Part model, mm, in its own coordinate system. A direction names the side the tool comes from. Give positions to 0.01 mm unless a question says otherwise; leave off trailing zeros. Write each loop counter-clockwise with the first axis right and the second up, starting at its lowest first coordinate (ties: lowest second). Pieces come first, ordered by that corner, then holes. Notation, with made-up numbers: M -25,67.25 L 0,67.25 A22 ccw 0,74.25 Z; hole C 67.5,67.5 d7. An arc over 180 degrees is marked long. Use a Markdown table: item, result. Add a question column.
from build123d import *

# Parameters (mm, degrees)
SKETCH_1_R                = 77.5
EXTRUDE_1_DEPTH           = 35
SKETCH_2_R                = 15
CUT_EXTRUDE_1_DEPTH       = 116.05433499
CHAMFER_1_SIZE            = 1
HOLE_WIZARD_1_D           = 8
HOLE_WIZARD_1_CBORE_D     = 14
HOLE_WIZARD_1_CBORE_DEPTH = 9
PATTERN_CIRCULAR_1_COUNT  = 5
HOLE_WIZARD_M8_1_D        = 6.8
CUT_EXTRUDE_2_DEPTH       = 24
FILLET_1_R                = 5


with BuildPart() as part:
    # 草图1 → 凸台-拉伸1 (new body)
    with BuildSketch(Plane.XY):
        Circle(SKETCH_1_R)
    extrude(amount=EXTRUDE_1_DEPTH)

    # 草图2 → 切除-拉伸1 (cut, through all)
    with BuildSketch(Plane.XY.offset(35)):
        with Locations((-4, -57)):
            Circle(SKETCH_2_R)
    extrude(amount=-CUT_EXTRUDE_1_DEPTH, mode=Mode.SUBTRACT)

    # 倒角1
    chamfer_1_edges = [part.edges().sort_by_distance(p)[0] for p in [
        (-19, -57, 0),
        (-19, -57, 35),
    ]]
    chamfer(chamfer_1_edges, length=CHAMFER_1_SIZE)

    # 孔1 (through all)
    with Locations(Plane(origin=(0, 0, 0), x_dir=(1, 0, 0), z_dir=(0, 0, -1))):
        with Locations((0, -70)):
            hole_wizard_1 = CounterBoreHole(HOLE_WIZARD_1_D / 2, HOLE_WIZARD_1_CBORE_D / 2, HOLE_WIZARD_1_CBORE_DEPTH)

    # 阵列(圆周)1: 孔1 ×5 about axis
    pattern_circular_1_axis = Axis((0, 0, 0), (0, 0, 1))
    for i in range(1, PATTERN_CIRCULAR_1_COUNT):
        add(hole_wizard_1.rotate(pattern_circular_1_axis, i * 360 / PATTERN_CIRCULAR_1_COUNT), mode=Mode.SUBTRACT)

    # M8 螺纹孔1 (through all)
    with Locations(Plane.XY.offset(35)):
        with Locations((-56.631189606, 41.14496766), (56.631189606, -41.14496766)):
            Hole(HOLE_WIZARD_M8_1_D / 2)

    # 草图7 → 切除-拉伸2 (cut)
    with BuildSketch(Plane.XY.offset(35)):
        with BuildLine():
            ThreePointArc((57.446485936, 30.412189227), (38.206041399, 52.586104634), (11.171770317, 64.032738095))
            ThreePointArc((11.171770317, 64.032738095), (8.869948511, 63.894555935), (6.87493558, 62.738095238))
            ThreePointArc((6.87493558, 62.738095238), (0, 60), (-6.87493558, 62.738095238))
            ThreePointArc((-6.87493558, 62.738095238), (-8.869948511, 63.894555935), (-11.171770317, 64.032738095))
            ThreePointArc((-11.171770317, 64.032738095), (-29.509382483, 57.915424072), (-45.236971481, 46.67565116))
            ThreePointArc((-45.236971481, 46.67565116), (-46.478156676, 44.732216765), (-46.715199498, 42.438466857))
            ThreePointArc((-46.715199498, 42.438466857), (-48.266255482, 35.665197857), (-53.856148227, 31.537723241))
            ThreePointArc((-53.856148227, 31.537723241), (-56.923660159, 29.004053529), (-57.170403739, 25.033130556))
            ThreePointArc((-57.170403739, 25.033130556), (-57.22394433, 18.084743619), (-61.791946226, 12.848685341))
            ThreePointArc((-61.791946226, 12.848685341), (-63.508298607, 11.308681301), (-64.351019707, 9.162219309))
            ThreePointArc((-64.351019707, 9.162219309), (-61.818673559, -20.086104634), (-46.67565116, -45.236971481))
            ThreePointArc((-46.67565116, -45.236971481), (-44.732216765, -46.478156676), (-42.438466857, -46.715199498))
            ThreePointArc((-42.438466857, -46.715199498), (-38.357298199, -47.027601789), (-34.743162658, -48.948944315))
            ThreePointArc((-34.743162658, -48.948944315), (-30.381779111, -49.971285841), (-26.951883464, -47.089851391))
            ThreePointArc((-26.951883464, -47.089851391), (-0.114506142, -32.303786981), (20.88609771, -54.616275863))
            ThreePointArc((20.88609771, -54.616275863), (23.401425614, -58.491437463), (28.01859369, -58.651158622))
            ThreePointArc((28.01859369, -58.651158622), (28.309318995, -58.511387422), (28.599347072, -58.37017515))
            ThreePointArc((28.599347072, -58.37017515), (30.380338596, -56.905406523), (31.314587418, -54.797170987))
            ThreePointArc((31.314587418, -54.797170987), (34.882784548, -48.834712026), (41.474548269, -46.636622251))
            ThreePointArc((41.474548269, -46.636622251), (45.174872479, -45.174872479), (46.636622251, -41.474548269))
            ThreePointArc((46.636622251, -41.474548269), (48.834712026, -34.882784548), (54.797170987, -31.314587418))
            ThreePointArc((54.797170987, -31.314587418), (56.905406523, -30.380338596), (58.37017515, -28.599347072))
            ThreePointArc((58.37017515, -28.599347072), (64.199742139, -10.168240228), (64.351019707, 9.162219309))
            ThreePointArc((64.351019707, 9.162219309), (63.508298607, 11.308681301), (61.791946226, 12.848685341))
            ThreePointArc((61.791946226, 12.848685341), (57.063390978, 18.541019662), (57.543002367, 25.925589906))
            ThreePointArc((57.543002367, 25.925589906), (58.026368949, 28.180325963), (57.446485936, 30.412189227))
        make_face()
    extrude(amount=-CUT_EXTRUDE_2_DEPTH, mode=Mode.SUBTRACT)

    # 圆角1
    fillet_1_edges = [part.edges().sort_by_distance(p)[0] for p in [
        (23.401425614, -58.491437463, 11),
        (-0.114506142, -32.303786981, 11),
        (-30.381779111, -49.971285841, 11),
        (-38.357298199, -47.027601789, 11),
        (-44.732216765, -46.478156676, 11),
        (-61.818673559, -20.086104634, 11),
        (-63.508298607, 11.308681301, 11),
        (-57.22394433, 18.084743619, 11),
        (-56.923660159, 29.004053529, 11),
        (-48.266255482, 35.665197857, 11),
        (-46.478156676, 44.732216765, 11),
        (-29.509382483, 57.915424072, 11),
        (-8.869948511, 63.894555935, 11),
        (0, 60, 11),
        (8.869948511, 63.894555935, 11),
        (38.206041399, 52.586104634, 11),
        (58.026368949, 28.180325963, 11),
        (57.063390978, 18.541019662, 11),
        (63.508298607, 11.308681301, 11),
        (64.199742139, -10.168240228, 11),
        (56.905406523, -30.380338596, 11),
        (48.834712026, -34.882784548, 11),
        (45.174872479, -45.174872479, 11),
        (34.882784548, -48.834712026, 11),
        (30.380338596, -56.905406523, 11),
        (28.309318995, -58.511387422, 11),
    ]]
    fillet(fillet_1_edges, radius=FILLET_1_R)


solid = part.part
1. Mould opens along Y. For faces 1 (the cylindrical face through (62.7, 22.63, 22.18)), 2 (the flat face through (-69, 25, 9)) say: released by +Y, released by -Y, zero draft, split by the parting line, or undercut.
2. Cut at A-A (z = 6). Give the number of separate pieces and of enclosed holes in the cut face, then the cut area to 3 significant figures.
3. Cut at B-B (y = 70). Write the cut outline in (x, z), then the cut area to 3 significant figures.
4. Drill centre lines: probe 1 along Y at (x, z) = (-14, 15.5) (3 decimals); probe 2 along Y at (x, z) = (-17.5, 14); probe 3 along Z at (x, y) = (43, 15.5). Where is each one in solid material? Low to high. Write a range as [from, to].
5. Flat gauge pins, fed straight in: pin 1 (12 mm diameter, centred on y = -59, z = 16.5, fed in from +X); pin 2 (3 mm diameter, centred on y = 4, z = 21, fed in from +X); pin 3 (1 mm diameter, centred on x = -23.5, y = -1, fed in from -Z); pin 4 (7 mm diameter, centred on x = 41, y = -54, fed in from -Z). Where does each tip first touch, or does it go through?
6. Tool access for faces 3 (the cylindrical face through (63.53, 11.28, 25.63)), 4 (the cylindrical face through (-56.189, 44.516, 17.255)), 5 (the flat face through (40, -61, 9)): list every direction of +Z, -Z, +X, -X, +Y, -Y with a clear straight run to the whole face (end or side of a thin tool).
A:
| question | item | result |
|---|---|---|
| 1 | face 1 | undercut |
| 1 | face 2 | undercut |
| 2 | separate pieces | 1 |
| 2 | enclosed holes | 8 |
| 2 | area | 17,300 mm² |
| 3 | outline | M -33.26,0 L -7,0 L -7,9 L -4,9 L -4,35 L -33.26,35 Z; M 4,9 L 7,9 L 7,0 L 33.26,0 L 33.26,35 L 4,35 Z |
| 3 | area | 1,990 mm² |
| 4 | probe 1 | y = [-76.225, -68.18], [-45.82, -34.06], [63.449, 76.225] |
| 4 | probe 2 | y = [-75.5, -63.54], [-50.46, -35.46], [62.17, 75.5] |
| 4 | probe 3 | z = [0, 11] |
| 5 | pin 1 | stops at x = 56.54 |
| 5 | pin 2 | stops at x = 77.46 |
| 5 | pin 3 | stops at z = 0 |
| 5 | pin 4 | stops at z = 9 |
| 6 | face 3 | +Z |
| 6 | face 4 | +Z, -Z |
| 6 | face 5 | -Z |
